The model under review builds one solid part; all positions refer to its coordinate system, in mm. A direction names the side the tool comes from. Round coordinates to 2 decimals unless told otherwise and drop trailing zeros. Order: outer loops, then holes, each group sorted by start corner. A loop starts at its lowest first (then second) coordinate and runs counter-clockwise, first axis right, second up. Notation, with made-up numbers: M -19.5,25.25 L -10.5,25.25 A13 cw -10.5,50.25 Z; hole C -29,52 d10. An arc over 180 degrees is marked long. Answer as a JSON object with one key per item and string values. Group by question number.
1. Mouldability with a two-part tool opening along X and no side actions: class faces 1 (the face through (175.512, 11, 144)), 2 (the face through (50, 13, 291.846)), 3 (the face through (178.052, 13, 144)), 4 (the face through (-81.308, 13, 148)) as released by +X, released by -X, zero draft, split by the parting line, or undercut.
2. Add section B-B on z = 236.5. State the section outline as (x, y) points, and give its area (3 significant figures).
3. Clearance check with a flat-ended pin moving along its axis: P1, Ø1.5, axis at x = 148.5, z = 81, coming from the -Y side. State where the tip first meets the part, or that it passes through.
4. To check wall thickness, follow probe 1 along X at (y, z) = (46, 114); probe 2 along Z at (x, y) = (159, 6); probe 3 along Y at (x, z) = (164.5, 42). State the ranges of each line that lie inside material, in increasing order. Write a range as [from, to].
5. Machinability: for faces 5 (the face through (47, 11, 2.54)), 6 (the face through (50, 51.665, 144)), which of the approach directions +Z, -Z, +X, -X, +Y, -Y give a long, thin tool a straight path to every point of the face, cutting with its end or side? Answer none if there is none.
6. Add section C-C on x = 44.5. State the section outline as (y, z) points, and give its area (3 significant figures).
7. Add section A-A on y = -8. State the section outline as (x, z) points.
```python
from build123d import *

# Parameters (mm, degrees)
F0_W     = 76.2264374644
F0_H     = 25.4088118672
F1_DEPTH = 113.792
F2_DEPTH = 183.134
F3_DEPTH = 178.054
F4_DEPTH = 53.594
F5_T     = -2.54


with BuildPart() as f1:
    # F0 (on Top) → F1 (new body)
    with BuildSketch(Plane.XY):
        with Locations((-43.1949794292, 38.960184902)):
            Rectangle(F0_W, F0_H)
    extrude(amount=F1_DEPTH)

    # F2 (add): a face of the model
    f2_faces = [f1.faces().sort_by_distance(p)[0] for p in [
        (-5.0817606971, 38.960184902, 56.896),
    ]]
    extrude(f2_faces, amount=F2_DEPTH)

    # F3 (add): a face of the model
    f3_faces = [f1.faces().sort_by_distance(p)[0] for p in [
        (48.3720205708, 38.960184902, 113.792),
    ]]
    extrude(f3_faces, amount=F3_DEPTH)

    # F4 (add): a face of the model
    f4_faces = [f1.faces().sort_by_distance(p)[0] for p in [
        (48.3720205708, 26.2557789683, 145.923),
    ]]
    extrude(f4_faces, amount=F4_DEPTH)

    # F5
    f5_openings = [f1.faces().sort_by_distance(p)[0] for p in [
        (48.372021, -27.338221, 145.923),
    ]]
    offset(amount=F5_T, openings=f5_openings)


solid = f1.part
```
Recorded:
{
 "1": {"face 1": "undercut", "face 2": "zero draft", "face 3": "released by +X", "face 4": "released by -X"},
 "2": {"outline": "M -81.31,-27.34 L -78.77,-27.34 L -78.77,49.12 L 175.51,49.12 L 175.51,-27.34 L 178.05,-27.34 L 178.05,51.66 L -81.31,51.66 Z", "area": "1,050 mm²"},
 "3": {"P1": "stops at y = 49.12"},
 "4": {"probe 1": "x = [-81.31, -78.77], [175.51, 178.05]", "probe 2": "z = [0, 2.54], [289.31, 291.85]", "probe 3": "y = [49.12, 51.66]"},
 "5": {"face 5": "-Y", "face 6": "+Z, -Z, +X, -X, +Y"},
 "6": {"outline": "M -27.34,0 L 51.66,0 L 51.66,291.85 L -27.34,291.85 L -27.34,289.31 L 49.12,289.31 L 49.12,2.54 L -27.34,2.54 Z", "area": "1,130 mm²"},
 "7": {"outline": "M -81.31,0 L 178.05,0 L 178.05,291.85 L -81.31,291.85 Z; hole M -78.77,2.54 L 175.51,2.54 L 175.51,289.31 L -78.77,289.31 Z"}
}
